Verification items for the finished model (mm, model axes). A direction names the side the tool comes from. Coordinates: 2 decimals unless noted, no trailing zeros. Write each loop counter-clockwise with the first axis right and the second up, starting at its lowest first coordinate (ties: lowest second). Pieces come first, ordered by that corner, then holes. Notation, with made-up numbers: (19.25, 43.5) -> (65.25, 43.5) arc R32 cw to (65.25, 80.5) -> close; hole circle Ø3 at (89, -27.5). An arc over 180 degrees is marked (long way). Answer in a Markdown table with one row per item.
```python
from build123d import *

# Parameters (mm, degrees)
F2_R    = 5.08
F3_SIZE = 7.62


with BuildPart() as f1:
    # F0 (on Front) → F1 (revolve)
    with BuildSketch(Plane.XZ):
        Polygon((-43.622624, 52.801218), (-56.252953, 52.801218), (-55.691604, -39.259836), (0, -39.259836), (0, -26.629508), (-38.289819, -26.629508), (-38.289819, 38.767517), align=None)
    revolve(axis=Axis((0, 0, -32.944672), (0, 0, -1)))

    # F2
    f2_edges = [f1.edges().sort_by_distance(p)[0] for p in [
        (43.622624, 0, 52.801218),
    ]]
    fillet(f2_edges, radius=F2_R)

    # F3
    f3_edges = [f1.edges().sort_by_distance(p)[0] for p in [
        (55.691604, 0, -39.259836),
    ]]
    chamfer(f3_edges, length=F3_SIZE)


solid = f1.part
```
1. Tool access check on faces 4 (the flat face through (-13, -46, 52.801)), 5 (the flat face through (-1, 1, -26.63)). Record the directions out of +Z, -Z, +X, -X, +Y, -Y that give a thin tool (end or side, any length) a straight path to the whole face; none if there is none.
Geometry says:
| item | result |
|---|---|
| face 4 | +Z, +X, -X, +Y, -Y |
| face 5 | +Z |
2. Depth check by flat-ended pin: P1, Ø8, axis at x = -15.5, z = -26.5, coming from the -Y side; P2, Ø8, axis at y = 29, z = -5, coming from the -X side; P3, Ø4, axis at y = 26.5, z = -5.5, coming from the -X side. Enter the tip coordinate at first touch or a pass-through.
Geometry says:
| item | result |
|---|---|
| P1 | y = -54.57 |
| P2 | x = -50 |
| P3 | x = -50.24 |
3. Section check B-B, the plane z = -11. Record the boundary of the cut face in (x, y), plus the area to 3 significant figures.
Geometry says:
| item | result |
|---|---|
| outline | circle Ø111.73 at (0, 0); hole circle Ø76.58 at (0, 0) |
| area | 5,200 mm^2 |
4. Section check A-A, the plane z = -21.5. Record the boundary of the cut face in (x, y), plus the area to 3 significant figures.
Geometry says:
| item | result |
|---|---|
| outline | circle Ø111.6 at (0, 0); hole circle Ø76.58 at (0, 0) |
| area | 5,180 mm^2 |
5. Thickness scan on line 1 (Y direction, x = 0, z = 18); line 2 (Y direction, x = 21, z = 30.5); line 3 (X direction, y = -35.5, z = 4). Record the ranges inside material, lowest first. Write a range as from..to.
Geometry says:
| item | result |
|---|---|
| line 1 | -56.04..-38.29, 38.29..56.04 |
| line 2 | -52.04..-32.02, 32.02..52.04 |
| line 3 | -43.25..-14.35, 14.35..43.25 |
6. Mould release check, pull along X, two halves, no side actions. Record for faces 1 (the conical face through (12.14, -54.66, 9.99)), 2 (the flat face through (1, 1, -39.26)), 3 (the cylindrical face through (-36.52, 11.5, 6.53)): released by +X, released by -X, zero draft, split by the parting line, or undercut.
Geometry says:
| item | result |
|---|---|
| face 1 | split by the parting line |
| face 2 | zero draft |
| face 3 | undercut |
